The model under review builds one solid part; all positions refer to its coordinate system, in mm. A direction names the side the tool comes from. Coordinates: 2 decimals unless noted, no trailing zeros. Order: outer loops, then holes, each group sorted by start corner. A loop starts at its lowest first (then second) coordinate and runs counter-clockwise, first axis right, second up. Notation, with made-up numbers: M -12,70.5 L 5,70.5 A16 cw 5,95.5 Z; hole C -37,-37 d4. An arc over 180 degrees is marked long. Answer in a Markdown table with one row per item.
from build123d import *

# Parameters (mm, degrees)
SKETCH1_W           = 609.6
SKETCH1_H           = 393.7
BOSS_EXTRUDE1_DEPTH = 6.35
SKETCH2_W           = 609.6
SKETCH2_H           = 215.9
BOSS_EXTRUDE2_DEPTH = 50.8


with BuildPart() as part:
    # Sketch1 → Boss-Extrude1 (new body)
    with BuildSketch(Plane(origin=(0, 0, 0), x_dir=(1, 0, 0), z_dir=(0, 1, 0))):
        with Locations((304.8, 196.85)):
            Rectangle(SKETCH1_W, SKETCH1_H)
        with BuildLine():
            Line((587.8, 32.05), (587.8, 17.05))
            ThreePointArc((587.8, 17.05), (584.8, 14.05), (581.8, 17.05))
            Line((581.8, 17.05), (581.8, 32.05))
            ThreePointArc((581.8, 32.05), (584.8, 35.05), (587.8, 32.05))
        make_face(mode=Mode.SUBTRACT)
        with BuildLine():
            Line((527.8, 32.05), (527.8, 17.05))
            ThreePointArc((527.8, 17.05), (524.8, 14.05), (521.8, 17.05))
            Line((521.8, 17.05), (521.8, 32.05))
            ThreePointArc((521.8, 32.05), (524.8, 35.05), (527.8, 32.05))
        make_face(mode=Mode.SUBTRACT)
        with BuildLine():
            Line((467.8, 32.05), (467.8, 17.05))
            ThreePointArc((467.8, 17.05), (464.8, 14.05), (461.8, 17.05))
            Line((461.8, 17.05), (461.8, 32.05))
            ThreePointArc((461.8, 32.05), (464.8, 35.05), (467.8, 32.05))
        make_face(mode=Mode.SUBTRACT)
        with BuildLine():
            Line((407.8, 32.05), (407.8, 17.05))
            ThreePointArc((407.8, 17.05), (404.8, 14.05), (401.8, 17.05))
            Line((401.8, 17.05), (401.8, 32.05))
            ThreePointArc((401.8, 32.05), (404.8, 35.05), (407.8, 32.05))
        make_face(mode=Mode.SUBTRACT)
        with BuildLine():
            Line((347.8, 32.05), (347.8, 17.05))
            ThreePointArc((347.8, 17.05), (344.8, 14.05), (341.8, 17.05))
            Line((341.8, 17.05), (341.8, 32.05))
            ThreePointArc((341.8, 32.05), (344.8, 35.05), (347.8, 32.05))
        make_face(mode=Mode.SUBTRACT)
        with BuildLine():
            Line((287.8, 32.05), (287.8, 17.05))
            ThreePointArc((287.8, 17.05), (284.8, 14.05), (281.8, 17.05))
            Line((281.8, 17.05), (281.8, 32.05))
            ThreePointArc((281.8, 32.05), (284.8, 35.05), (287.8, 32.05))
        make_face(mode=Mode.SUBTRACT)
        with BuildLine():
            Line((227.8, 32.05), (227.8, 17.05))
            ThreePointArc((227.8, 17.05), (224.8, 14.05), (221.8, 17.05))
            Line((221.8, 17.05), (221.8, 32.05))
            ThreePointArc((221.8, 32.05), (224.8, 35.05), (227.8, 32.05))
        make_face(mode=Mode.SUBTRACT)
        with BuildLine():
            Line((167.8, 32.05), (167.8, 17.05))
            ThreePointArc((167.8, 17.05), (164.8, 14.05), (161.8, 17.05))
            Line((161.8, 17.05), (161.8, 32.05))
            ThreePointArc((161.8, 32.05), (164.8, 35.05), (167.8, 32.05))
        make_face(mode=Mode.SUBTRACT)
        with BuildLine():
            Line((107.8, 32.05), (107.8, 17.05))
            ThreePointArc((107.8, 17.05), (104.8, 14.05), (101.8, 17.05))
            Line((101.8, 17.05), (101.8, 32.05))
            ThreePointArc((101.8, 32.05), (104.8, 35.05), (107.8, 32.05))
        make_face(mode=Mode.SUBTRACT)
        with BuildLine():
            Line((47.8, 32.05), (47.8, 17.05))
            ThreePointArc((47.8, 17.05), (44.8, 14.05), (41.8, 17.05))
            Line((41.8, 17.05), (41.8, 32.05))
            ThreePointArc((41.8, 32.05), (44.8, 35.05), (47.8, 32.05))
        make_face(mode=Mode.SUBTRACT)
        with BuildLine():
            Line((527.8, 376.65), (527.8, 361.65))
            ThreePointArc((527.8, 361.65), (524.8, 358.65), (521.8, 361.65))
            Line((521.8, 361.65), (521.8, 376.65))
            ThreePointArc((521.8, 376.65), (524.8, 379.65), (527.8, 376.65))
        make_face(mode=Mode.SUBTRACT)
        with BuildLine():
            Line((467.8, 376.65), (467.8, 361.65))
            ThreePointArc((467.8, 361.65), (464.8, 358.65), (461.8, 361.65))
            Line((461.8, 361.65), (461.8, 376.65))
            ThreePointArc((461.8, 376.65), (464.8, 379.65), (467.8, 376.65))
        make_face(mode=Mode.SUBTRACT)
        with BuildLine():
            Line((407.8, 376.65), (407.8, 361.65))
            ThreePointArc((407.8, 361.65), (404.8, 358.65), (401.8, 361.65))
            Line((401.8, 361.65), (401.8, 376.65))
            ThreePointArc((401.8, 376.65), (404.8, 379.65), (407.8, 376.65))
        make_face(mode=Mode.SUBTRACT)
        with BuildLine():
            Line((347.8, 376.65), (347.8, 361.65))
            ThreePointArc((347.8, 361.65), (344.8, 358.65), (341.8, 361.65))
            Line((341.8, 361.65), (341.8, 376.65))
            ThreePointArc((341.8, 376.65), (344.8, 379.65), (347.8, 376.65))
        make_face(mode=Mode.SUBTRACT)
        with BuildLine():
            Line((287.8, 376.65), (287.8, 361.65))
            ThreePointArc((287.8, 361.65), (284.8, 358.65), (281.8, 361.65))
            Line((281.8, 361.65), (281.8, 376.65))
            ThreePointArc((281.8, 376.65), (284.8, 379.65), (287.8, 376.65))
        make_face(mode=Mode.SUBTRACT)
        with BuildLine():
            Line((227.8, 376.65), (227.8, 361.65))
            ThreePointArc((227.8, 361.65), (224.8, 358.65), (221.8, 361.65))
            Line((221.8, 361.65), (221.8, 376.65))
            ThreePointArc((221.8, 376.65), (224.8, 379.65), (227.8, 376.65))
        make_face(mode=Mode.SUBTRACT)
        with BuildLine():
            Line((167.8, 376.65), (167.8, 361.65))
            ThreePointArc((167.8, 361.65), (164.8, 358.65), (161.8, 361.65))
            Line((161.8, 361.65), (161.8, 376.65))
            ThreePointArc((161.8, 376.65), (164.8, 379.65), (167.8, 376.65))
        make_face(mode=Mode.SUBTRACT)
        with BuildLine():
            Line((107.8, 376.65), (107.8, 361.65))
            ThreePointArc((107.8, 361.65), (104.8, 358.65), (101.8, 361.65))
            Line((101.8, 361.65), (101.8, 376.65))
            ThreePointArc((101.8, 376.65), (104.8, 379.65), (107.8, 376.65))
        make_face(mode=Mode.SUBTRACT)
        with BuildLine():
            Line((47.8, 376.65), (47.8, 361.65))
            ThreePointArc((47.8, 361.65), (44.8, 358.65), (41.8, 361.65))
            Line((41.8, 361.65), (41.8, 376.65))
            ThreePointArc((41.8, 376.65), (44.8, 379.65), (47.8, 376.65))
        make_face(mode=Mode.SUBTRACT)
        with BuildLine():
            Line((587.8, 376.65), (587.8, 361.65))
            ThreePointArc((587.8, 361.65), (584.8, 358.65), (581.8, 361.65))
            Line((581.8, 361.65), (581.8, 376.65))
            ThreePointArc((581.8, 376.65), (584.8, 379.65), (587.8, 376.65))
        make_face(mode=Mode.SUBTRACT)
        with BuildLine():
            Line((506.85, 209.125), (556.85, 209.125))
            ThreePointArc((556.85, 209.125), (559.6, 206.375), (556.85, 203.625))
            Line((556.85, 203.625), (506.85, 203.625))
            ThreePointArc((506.85, 203.625), (504.1, 206.375), (506.85, 209.125))
        make_face(mode=Mode.SUBTRACT)
        with BuildLine():
            Line((506.85, 190.075), (556.85, 190.075))
            ThreePointArc((556.85, 190.075), (559.6, 187.325), (556.85, 184.575))
            Line((556.85, 184.575), (506.85, 184.575))
            ThreePointArc((506.85, 184.575), (504.1, 187.325), (506.85, 190.075))
        make_face(mode=Mode.SUBTRACT)
    extrude(amount=BOSS_EXTRUDE1_DEPTH)

    # Sketch2 → Boss-Extrude2 (add)
    with BuildSketch(Plane.XZ):
        with Locations((304.8, 107.95)):
            Rectangle(SKETCH2_W, SKETCH2_H)
    extrude(amount=-BOSS_EXTRUDE2_DEPTH)


solid = part.part
(1) Take a section at B-B (y = 24.5). Write out the cut boundary in (x, z).
Report:
| item | result |
|---|---|
| outline | M 0,0 L 609.6,0 L 609.6,215.9 L 0,215.9 Z |
(2) Take a section at C-C (z = -303). Write out the cut boundary in (x, y), then the cut area to 3 significant figures.
Report:
| item | result |
|---|---|
| outline | M 0,0 L 609.6,0 L 609.6,6.35 L 0,6.35 Z |
| area | 3,870 mm^2 |
(3) To check wall thickness, follow line 1 (Y direction, x = 246, z = -170.5); line 2 (Z direction, x = 213, y = 42). State the ranges of each line that lie inside material, in increasing order. Write a range as [from, to].
Report:
| item | result |
|---|---|
| line 1 | [0, 6.35] |
| line 2 | [0, 215.9] |
(4) Insertion check: P1, Ø3, axis at x = 458.5, y = 44, coming from the -Z side; P2, Ø8, axis at x = 466.5, z = -253, coming from the +Y side; P3, Ø8, axis at y = 11.5, z = -39.5, coming from the -X side. Each pin has a flat end and moves straight along its axis. Give the tip position at first contact, or say it passes through.
Report:
| item | result |
|---|---|
| P1 | z = 0 |
| P2 | y = 6.35 |
| P3 | through |
(5) Machinability: for faces 1 (the flat face through (301, 50.8, 109)), 2 (the flat face through (301, 28, 0)), which of the approach directions +Z, -Z, +X, -X, +Y, -Y give a long, thin tool a straight path to every point of the face, cutting with its end or side? Answer none if there is none.
Report:
| item | result |
|---|---|
| face 1 | +Z, -Z, +X, -X, +Y |
| face 2 | -Z, +X, -X, +Y |
(6) Take a section at A-A (x = 148). Write out the cut boundary in (y, z), then the cut area to 3 significant figures.
Report:
| item | result |
|---|---|
| outline | M 0,-393.7 L 6.35,-393.7 L 6.35,0 L 50.8,0 L 50.8,215.9 L 0,215.9 Z |
| area | 13,500 mm^2 |
